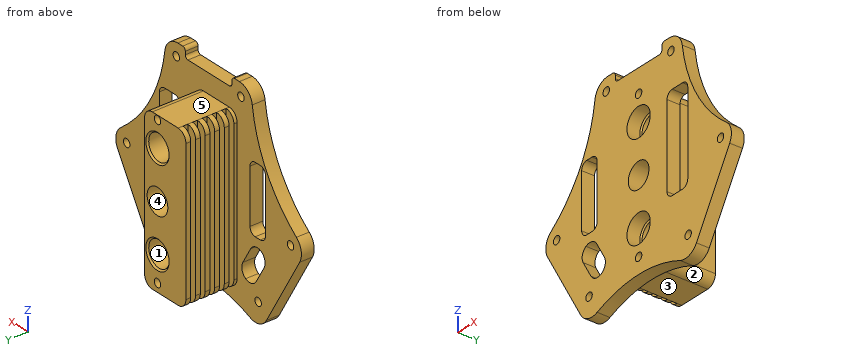
from build123d import *

# Parameters (mm, degrees)
EXTRUDE_1_DEPTH           = 4
FILLET_1_R                = 5
SKETCH_2_W                = 16
SKETCH_2_H                = 50
EXTRUDE_2_DEPTH           = 16
FILLET_2_R                = 3
SKETCH_3_W                = 6.925100322
SKETCH_3_H                = 1.5
CUT_EXTRUDE_1_DEPTH       = 70.527213361
SKETCH_4_W                = 8
SKETCH_4_H                = 30
CUT_EXTRUDE_2_DEPTH       = 52.527238457
FILLET_3_R                = 2
SKETCH_5_R                = 4
CUT_EXTRUDE_3_DEPTH       = 53.906108371
SKETCH_6_W                = 6
SKETCH_6_H                = 21
CUT_EXTRUDE_4_DEPTH       = 52.527238457
FILLET_4_R                = 2
SKETCH_7_R                = 4
CUT_EXTRUDE_5_DEPTH       = 53.906108371
CHAMFER_1_SIZE            = 0.5
M10X1_0_1_D               = 9
M10X1_0_1_DEPTH           = 4
M10X1_0_1_TIP             = 2.703872786
SKETCH_10_R               = 1
CUT_EXTRUDE_6_DEPTH       = 53.906108371
HOLE_WIZARD_M3_1_D        = 2.5
CUT_EXTRUDE_7_DEPTH       = 52.527238457
FILLET_5_R                = 3
SKETCH_17_W               = 18
SKETCH_17_H               = 3
CUT_EXTRUDE_10_DEPTH      = 4
SKETCH_18_R               = 1
CUT_EXTRUDE_11_DEPTH      = 52.527238457
HOLE_WIZARD_M3_3_D        = 2.5
PATTERN_CIRCULAR_14_COUNT = 3
FILLET_8_R                = 1


with BuildPart() as part:
    # 草圖1 → 填料-伸長1 (new body)
    with BuildSketch(Plane(origin=(0, 0, 0), x_dir=(1, 0, 0), z_dir=(0, 1, 0))):
        with BuildLine():
            Line((20, 33.341978046), (37.5, 3.031088913))
            ThreePointArc((37.5, 3.031088913), (22.496232709, -12.555193308), (16.5, -33.341978046))
            Line((16.5, -33.341978046), (-16.5, -33.341978046))
            ThreePointArc((-16.5, -33.341978046), (-22.496232709, -12.555193308), (-37.5, 3.031088913))
            Line((-37.5, 3.031088913), (-20, 33.341978046))
            ThreePointArc((-20, 33.341978046), (0, 27.982994197), (20, 33.341978046))
        make_face()
    extrude(amount=EXTRUDE_1_DEPTH)

    # 圓角1
    fillet_1_edges = [part.edges().sort_by_distance(p)[0] for p in [
        (20, 2, -33.341978046),
        (37.5, 2, -3.031088913),
        (16.5, 2, 33.341978046),
        (-16.5, 2, 33.341978046),
        (-37.5, 2, -3.031088913),
        (-20, 2, -33.341978046),
    ]]
    fillet(fillet_1_edges, radius=FILLET_1_R)

    # 草圖2 → 填料-伸長2 (add)
    with BuildSketch(Plane(origin=(0, 4, 0), x_dir=(1, 0, 0), z_dir=(0, 1, 0))):
        with Locations((-3, 0.658021954)):
            Rectangle(SKETCH_2_W, SKETCH_2_H)
    extrude(amount=EXTRUDE_2_DEPTH)

    # 圓角2
    fillet_2_edges = [part.edges().sort_by_distance(p)[0] for p in [
        (-11, 12, -25.658021954),
        (-11, 12, 24.341978046),
        (5, 12, 24.341978046),
        (5, 12, -25.658021954),
    ]]
    fillet(fillet_2_edges, radius=FILLET_2_R)

    # 草圖3 → 除料-伸長1 (cut, through all)
    with BuildSketch(Plane.XY.offset(24.341978046)):
        with Locations((-11.462550161, 17.75)):
            Rectangle(SKETCH_3_W, SKETCH_3_H)
        with Locations((-11.462550161, 14.75)):
            Rectangle(SKETCH_3_W, SKETCH_3_H)
        with Locations((-11.462550161, 11.75)):
            Rectangle(SKETCH_3_W, SKETCH_3_H)
        with Locations((-11.462550161, 8.75)):
            Rectangle(SKETCH_3_W, SKETCH_3_H)
        with Locations((-11.462550161, 5.75)):
            Rectangle(SKETCH_3_W, SKETCH_3_H)
    extrude(amount=-CUT_EXTRUDE_1_DEPTH, mode=Mode.SUBTRACT)

    # 草圖4 → 除料-伸長2 (cut, through all)
    with BuildSketch(Plane(origin=(0, 4, 0), x_dir=(1, 0, 0), z_dir=(0, 1, 0))):
        with Locations((15, -3.341978046)):
            Rectangle(SKETCH_4_W, SKETCH_4_H)
    extrude(amount=-CUT_EXTRUDE_2_DEPTH, mode=Mode.SUBTRACT)

    # 圓角3
    fillet_3_edges = [part.edges().sort_by_distance(p)[0] for p in [
        (11, 2, 18.341978046),
        (11, 2, -11.658021954),
        (19, 2, -11.658021954),
        (19, 2, 18.341978046),
    ]]
    fillet(fillet_3_edges, radius=FILLET_3_R)

    # 草圖5 → 除料-伸長3 (cut, through all)
    with BuildSketch(Plane(origin=(0, 20, 0), x_dir=(1, 0, 0), z_dir=(0, 1, 0))):
        with Locations(Location((0, 0, 0), (0, 0, 270))):
            Circle(SKETCH_5_R)
    extrude(amount=-CUT_EXTRUDE_3_DEPTH, mode=Mode.SUBTRACT)

    # 草圖6 → 除料-伸長4 (cut, through all)
    with BuildSketch(Plane(origin=(0, 4, 0), x_dir=(1, 0, 0), z_dir=(0, 1, 0))):
        with Locations((-19, -2.841978046)):
            Rectangle(SKETCH_6_W, SKETCH_6_H)
    extrude(amount=-CUT_EXTRUDE_4_DEPTH, mode=Mode.SUBTRACT)

    # 圓角4
    fillet_4_edges = [part.edges().sort_by_distance(p)[0] for p in [
        (-22, 2, 13.341978046),
        (-22, 2, -7.658021954),
        (-16, 2, -7.658021954),
        (-16, 2, 13.341978046),
    ]]
    fillet(fillet_4_edges, radius=FILLET_4_R)

    # 草圖7 → 除料-伸長5 (cut, through all)
    with BuildSketch(Plane.XZ):
        with Locations(Location((0, 15, 0), (0, 0, 270))):
            Circle(SKETCH_7_R)
        with Locations(Location((0, -15, 0), (0, 0, 270))):
            Circle(SKETCH_7_R)
    extrude(amount=-CUT_EXTRUDE_5_DEPTH, mode=Mode.SUBTRACT)

    # 導角1
    chamfer_1_edges = [part.edges().sort_by_distance(p)[0] for p in [
        (0, 20, 19),
        (0, 20, -11),
    ]]
    chamfer(chamfer_1_edges, length=CHAMFER_1_SIZE)

    # M10x1.0 螺紋孔1
    with Locations(Plane(origin=(0, 0, 0), x_dir=(-1, 0, 0), z_dir=(0, -1, 0))):
        with Locations((0, 15), (0, -15)):
            Hole(M10X1_0_1_D / 2, depth=M10X1_0_1_DEPTH)
            with Locations((0, 0, -(M10X1_0_1_DEPTH + M10X1_0_1_TIP / 2))):  # 118° drill point
                Cone(0, M10X1_0_1_D / 2, M10X1_0_1_TIP, mode=Mode.SUBTRACT)

    # 草圖10 → 除料-伸長6 (cut, through all)
    with BuildSketch(Plane.XZ):
        with Locations(Location((0, 23, 0), (0, 0, 270))):
            Circle(SKETCH_10_R)
        with Locations(Location((0, -23, 0), (0, 0, 270))):
            Circle(SKETCH_10_R)
    extrude(amount=-CUT_EXTRUDE_6_DEPTH, mode=Mode.SUBTRACT)

    # M3 螺紋孔1 (through all)
    with Locations(Plane(origin=(0, 20, 23), x_dir=(0, 0, 1), z_dir=(0, 1, 0))):
        with Locations((0, 0), (-46, 0)):
            Hole(HOLE_WIZARD_M3_1_D / 2)

    # 草圖12 → 除料-伸長7 (cut, through all)
    with BuildSketch(Plane(origin=(0, 4, 0), x_dir=(1, 0, 0), z_dir=(0, 1, 0))):
        Polygon((-16.932476545, 22.655084524), (-22.932476545, 12.262779678), (-17.736324122, 9.262779678), (-11.736324122, 19.655084524), align=None)
    extrude(amount=-CUT_EXTRUDE_7_DEPTH, mode=Mode.SUBTRACT)

    # 圓角5
    fillet_5_edges = [part.edges().sort_by_distance(p)[0] for p in [
        (-11.736324122, 2, -19.655084524),
        (-17.736324122, 2, -9.262779678),
        (-22.932476545, 2, -12.262779678),
        (-16.932476545, 2, -22.655084524),
    ]]
    fillet(fillet_5_edges, radius=FILLET_5_R - 0.0001)  # a hair under: the kernel refuses the full size

    # 草圖17 → 除料-伸長10 (cut)
    with BuildSketch(Plane.XZ):
        with Locations((0, 31.841978046)):
            Rectangle(SKETCH_17_W, SKETCH_17_H)
    extrude(amount=-CUT_EXTRUDE_10_DEPTH, mode=Mode.SUBTRACT)

    # 草圖18 → 除料-伸長11 (cut, through all)
    with BuildSketch(Plane(origin=(0, 4, 0), x_dir=(1, 0, 0), z_dir=(0, 1, 0))):
        with Locations(Location((-12.5, -29.341978046, 0), (0, 0, 270))):
            Circle(SKETCH_18_R)
        with Locations(Location((12.5, -29.341978046, 0), (0, 0, 270))):
            Circle(SKETCH_18_R)
    cut_extrude_11 = extrude(amount=-CUT_EXTRUDE_11_DEPTH, mode=Mode.SUBTRACT)

    # M3 螺紋孔3 (through all)
    with Locations(Plane(origin=(-12.5, 4, 29.341978046), x_dir=(0, 0, 1), z_dir=(0, 1, 0))):
        with Locations((0, 0), (0, 25)):
            hole_wizard_m3_3 = Hole(HOLE_WIZARD_M3_3_D / 2)

    # 環狀複製排列14: 除料-伸長11, M3 螺紋孔3 ×3 about axis
    pattern_circular_14_axis = Axis((0, 0, 0), (0, 1, 0))
    add([cut_extrude_11.rotate(pattern_circular_14_axis, i * 360 / PATTERN_CIRCULAR_14_COUNT) for i in range(1, PATTERN_CIRCULAR_14_COUNT)], mode=Mode.SUBTRACT)
    add([hole_wizard_m3_3.rotate(pattern_circular_14_axis, i * 360 / PATTERN_CIRCULAR_14_COUNT) for i in range(1, PATTERN_CIRCULAR_14_COUNT)], mode=Mode.SUBTRACT)

    # 圓角8
    fillet_8_edges = [part.edges().sort_by_distance(p)[0] for p in [
        (-9, 2, 30.341978046),
        (-9, 2, 33.341978046),
        (9, 2, 33.341978046),
        (9, 2, 30.341978046),
    ]]
    fillet(fillet_8_edges, radius=FILLET_8_R)


solid = part.part
Verification items for the finished model (mm, model axes). Face numbers are marked on the shaded views. A direction names the side the tool comes from. Coordinates: 2 decimals unless noted, no trailing zeros. Order: outer loops, then holes, each group sorted by start corner. A loop starts at its lowest first (then second) coordinate and runs counter-clockwise, first axis right, second up. Notation, with made-up numbers: M 16,66 L 45,66 A28 cw 45,92 Z; hole C 3.25,83 d1. An arc over 180 degrees is marked long. One line per item, written item: value. Start each with the question number.
Item 1: Sectioned sample at C-C (x = -26). Enter the section's corners in (y, z), then the cut area to 3 significant figures.
Item 2: Scan lines: probe 1 along Y at (x, z) = (-9, 20); probe 2 along X at (y, z) = (1.25, -11); probe 3 along X at (y, z) = (1.25, -24.5). Record each from-to range of solid material in increasing order.
Item 3: Mould release check, pull along X, two halves, no side actions. Record for the marked faces 1, 2 and 3: released by +X, released by -X, zero draft, split by the parting line, or undercut.
Item 4: Sectioned sample at A-A (z = -13). Count the separate pieces of the cut face and the enclosed holes in it, then the cut area to 3 significant figures.
Item 5: Access from +Z, -Z, +X, -X, +Y, -Y to the whole of each face (thin tool, end or side, straight path). Record for the marked faces 4 and 5.
Item 6: Sectioned sample at B-B (z = 27). Enter the section's corners in (x, y).
Item 7: Gauge pin test, flat ends, axial feed: pin 1 (2 mm diameter, centred on x = -6.5, y = 12.5, fed in from -Z); pin 2 (0.8 mm diameter, centred on y = 1, z = 32, fed in from +X); pin 3 (4.5 mm diameter, centred on x = 3, y = 1.5, fed in from +Z). Record the tip position at first contact, or that the pin passes through.
Conclusion:
1. outline: M 0,-22.95 L 4,-22.95 L 4,7.36 L 0,7.36 Z
1. area: 121 mm^2
2. probe 1: y = 0 to 5, 6.5 to 8, 9.5 to 11, 12.5 to 14, 15.5 to 17, 18.5 to 20
2. probe 2: x = -32.9 to -20.69, -16.98 to -2.06, 2.06 to 11.52, 18.48 to 32.9
2. probe 3: x = -25.1 to -19.92, -18.41 to 18.41, 19.92 to 25.1
3. face 1: undercut
3. face 2: released by +X
3. face 3: zero draft
4. separate pieces: 3
4. enclosed holes: 0
4. area: 319 mm^2
5. face 4: +Y, -Y
5. face 5: +Z, +X, -X, +Y
6. outline: M -17.19,0 L 17.19,0 L 17.19,4 L -17.19,4 Z
7. pin 1: stops at z = -25.66
7. pin 2: stops at x = 15.71
7. pin 3: stops at z = 30.34
